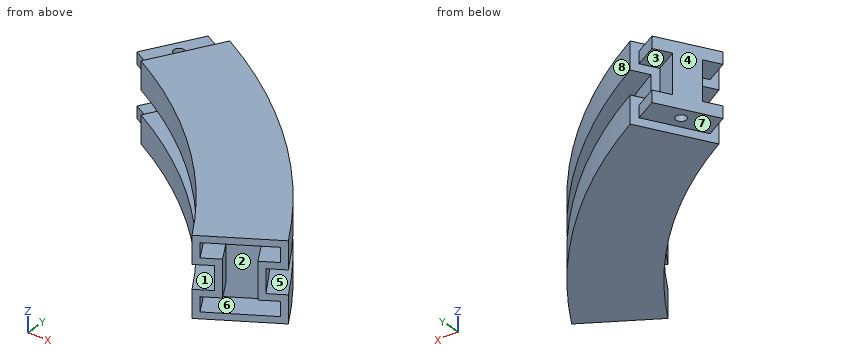
Autodesk Inventor part; units mm, degrees
ref_plane "Work Plane1" through (0, 50, 0) normal (0, 1, 0) x (-1, 0, 0)
ref_plane "Work Plane2" through (0, 0, -79) normal (0, 0, 1) x (1, 0, 0)
ref_plane "Work Plane3" through (-40, 45, 40) normal (0, -1, 0) x (1, 0, 0)
sketch "Sketch2" plane through (0, 0, 0) normal (0, 1, 0) x (-1, 0, 0)
  line L0 (15, 15) -> (-15, 15)
  line L1 (-15, -15) -> (15, -15)
  line L2 (15, 4.5) -> (8, 4.5)
  line L3 (8, 4.5) -> (8, -4.5)
  line L4 (8, -4.5) -> (15, -4.5)
  line L5 (-15, 4.5) -> (-8, 4.5)
  line L6 (-8, 4.5) -> (-8, -4.5)
  line L7 (-8, -4.5) -> (-15, -4.5)
  line L8 (15, -15) -> (15, -4.5)
  line L9 (15, 4.5) -> (15, 15)
  line L10 (-15, 15) -> (-15, 4.5)
  line L11 (-15, -4.5) -> (-15, -15)
  point P0 (0, 0)
  dimension "d18" = 9
  dimension "d19" = 7
  dimension "d21" = 16
  dimension "d22" = 30
  dimension "d23" = 15
  dimension "d24" = 4.5
  dimension "d25" = 8
sketch "Sketch6" plane through (0, 0, 0) normal (0, 0, 1) x (1, 0, 0)
  arc A0 (0, 0) -> (-110, 190.5256) centre (-220, 0) ccw
  line L0 (-220, 0) -> (-110, 190.5256) construction
  line L1 (-220, 0) -> (0, 0) construction
  dimension "d41" = 220
  dimension "d42" = 60
  dimension "d43" = 220
  dimension "d44" = 0
sweep "Sweep2" add profiles "Sketch2" path "Sketch6"
sketch "Sketch7" plane through (-102.5, 203.516, 4.5) normal (-0.8660254, 0.5, 0) x (0, 0, 1)
  line L0 (-16.5, -3) -> (-12, -3)
  line L1 (-12, -3) -> (-12, -10)
  line L2 (-12, -10) -> (3, -10)
  line L3 (3, -10) -> (3, -3)
  line L4 (3, -3) -> (7.5, -3)
  line L5 (7.5, -3) -> (7.5, -27)
  line L6 (7.5, -27) -> (3, -27)
  line L7 (3, -27) -> (3, -20)
  line L8 (3, -20) -> (-12, -20)
  line L9 (-12, -20) -> (-12, -27)
  line L10 (-12, -27) -> (-16.5, -27)
  line L11 (-16.5, -27) -> (-16.5, -3)
  line L12 (-19.5, 0) -> (-19.5, -30)
  line L13 (-9, -7) -> (-9, 0)
  line L14 (0, 0) -> (0, -7)
  line L15 (10.5, -30) -> (10.5, 0)
  line L16 (-19.5, -30) -> (-9, -30)
  line L17 (-9, 0) -> (-19.5, 0)
  line L18 (0, -30) -> (10.5, -30)
  line L19 (-9, -23) -> (0, -23)
  line L20 (0, -7) -> (-9, -7)
  point P0 (-4.5, -125)
  point P1 (-14.25, 0)
  dimension "d47" = 3
  dimension "d48" = 3
  dimension "d49" = 3
  dimension "d50" = 3
  dimension "d51" = 3
  dimension "d52" = 3
  dimension "d53" = 3
  dimension "d54" = 3
  dimension "d55" = 3
extrude "Extrusion3" add sketch "Sketch7" along normal blind 10
sketch "Sketch8" plane through (-116, 180.1333, -12) normal (0, 0, -1) x (-0.8660254, 0.5, 0)
  circle A0 centre (5, 12) radius 2
  line L0 (0, 0) -> (10, 0)
  line L1 (10, 24) -> (10, 0)
  point P0 (-190.5256, -98)
  dimension "d58" = 4
  dimension "d59" = 12
  dimension "d60" = 5
extrude "Extrusion4" cut sketch "Sketch8" against normal through all
sketch "Sketch9" plane through (0, 0, 0) normal (0, 1, 0) x (-1, 0, 0)
  line L0 (-40, 40) -> (40, 40)
  line L1 (40, 40) -> (40, -40)
  line L2 (40, -40) -> (-40, -40)
  line L3 (-40, -40) -> (-40, 40)
  point P0 (0, 0)
  dimension "d63" = 80
  dimension "d64" = 80
  dimension "d65" = 40
  dimension "d66" = 40
ref_plane "Work Plane1" through (0, 50, 0) normal (0, 1, 0) x (-1, 0, 0)
sketch "Sketch10" plane through (0, 50, 0) normal (0, 1, 0) x (-1, 0, 0)
  line L0 (-9.6, 15) -> (21.4, 15)
  line L1 (21.4, 15) -> (21.4, -15)
  line L2 (21.4, -15) -> (-9.6, -15)
  line L3 (-9.6, -15) -> (-9.6, 15)
  point P0 (0, 0)
  dimension "d68" = 30
  dimension "d69" = 9.6
  dimension "d70" = 15
  dimension "d71" = 31
loft "Loft1" add profiles "Sketch9", "Sketch10"
ref_plane "Work Plane2" through (0, 0, -79) normal (0, 0, 1) x (1, 0, 0)
sketch "Sketch11" plane through (0, 0, -79) normal (0, 0, 1) x (1, 0, 0)
  line L0 (50, -5) -> (-129.034, -5)
  line L1 (-129.034, -5) -> (-129.034, 135)
  line L2 (-129.034, 135) -> (-90, 202.6089)
  line L3 (-90, 202.6089) -> (50, 95)
  line L4 (50, -5) -> (50, 95)
  point P0 (0, 0)
  dimension "d77" = 100
  dimension "d79" = 140
  dimension "d80" = 67.6089
  dimension "d81" = 140
  dimension "d82" = 150
  dimension "d83" = 50
  dimension "d86" = 5
extrude "Extrusion5" [suppressed]
sketch "Sketch12" plane through (-40, 0, 40) normal (0, -1, 0) x (1, 0, 0)
  line L0 (70, -70) -> (10, -70)
  line L1 (10, -70) -> (10, -10)
  line L2 (10, -10) -> (70, -10)
  line L3 (70, -10) -> (70, -70)
  line L4 (0, 0) -> (0, -80)
  line L5 (0, -80) -> (80, -80)
  line L6 (80, -80) -> (80, 0)
  line L7 (80, 0) -> (0, 0)
  point P0 (40, -40)
  dimension "d87" = 10
  dimension "d88" = 10
  dimension "d89" = 10
  dimension "d90" = 10
ref_plane "Work Plane3" through (-40, 45, 40) normal (0, -1, 0) x (1, 0, 0)
sketch "Sketch14" plane through (-40, 45, 40) normal (0, -1, 0) x (1, 0, 0)
  line L0 (40.5, -40.5) -> (39.5, -40.5)
  line L1 (39.5, -40.5) -> (39.5, -39.5)
  line L2 (39.5, -39.5) -> (40.5, -39.5)
  line L3 (40.5, -39.5) -> (40.5, -40.5)
  line L4 (80, 0) -> (0, 0)
  line L5 (0, 0) -> (0, -80)
  point P0 (40, -40)
  point P1 (0, -40)
  dimension "d95" = 1
  dimension "d96" = 1
  dimension "d97" = 39.5
  dimension "d98" = 39.5
loft "Loft2" cut profiles "Sketch12", "Sketch14" contours L0 L1 L2 L3 / all
ref_plane "Work Plane4" through (9.6, 50, -45) normal (0, 0, -1) x (-1, 0, 0)
sketch "Sketch15" plane through (9.6, 50, -45) normal (0, 0, -1) x (-1, 0, 0)
  line L0 (-71.3683, -50) -> (104.0101, -50)
  line L1 (229.6, -50) -> (-99.4897, 140)
  line L2 (-99.4897, 140) -> (-99.4897, -50)
  line L3 (-99.4897, -50) -> (-71.3683, -50)
  line L4 (229.6, -50) -> (104.0101, -50)
  point P0 (9.6, -50)
  dimension "d104" = 220
  dimension "d105" = 30
  dimension "d107" = 190
extrude "Extrusion6" cut sketch "Sketch15" against normal through all
sketch "Sketch16" plane through (-42.4648, 102.5, -15) normal (0.5, -0.8660254, 0) x (0.8660254, 0.5, 0)
  line L0 (27.5, 27.5) -> (27.5, 22)
  line L1 (27.5, 22) -> (20.5, 22)
  line L2 (20.5, 22) -> (20.5, 8)
  line L3 (23, 10.5) -> (-7.5462, 10.5)
  line L4 (20.5, 8) -> (27.5, 8)
  line L5 (27.5, 8) -> (27.5, 2.5)
  line L6 (27.5, 2.5) -> (2.5, 2.5)
  line L7 (2.5, 2.5) -> (2.5, 8)
  line L8 (2.5, 8) -> (9.5, 8)
  line L9 (9.5, 8) -> (9.5, 22)
  line L10 (9.5, 22) -> (2.5, 22)
  line L11 (2.5, 27.5) -> (27.5, 27.5)
  line L12 (2.5, 22) -> (2.5, 27.5)
  line L13 (0, 30) -> (30, 30)
  line L14 (0, 19.5) -> (0, 30)
  line L15 (7, 19.5) -> (0, 19.5)
  line L16 (7, 10.5) -> (7, 19.5)
  line L17 (30, 0) -> (0, 0)
  line L18 (30, 10.5) -> (30, 0)
  line L19 (23, 19.5) -> (23, 10.5)
  point P0 (-14.4744, 15)
  dimension "d110" = 2.5
  dimension "d111" = 2.5
  dimension "d112" = 2.5
  dimension "d113" = 2.5
  dimension "d114" = 2.5
  dimension "d115" = 2.5
  dimension "d116" = 2.5
  dimension "d117" = 2.5
extrude "Extrusion7" cut sketch "Sketch16" against normal blind 10
properties part number "LightRail_endSection"
Source: CAD feature listing. Evaluate the final solid. Frame: model axes, mm. Face numbers are marked on the shaded views. A direction names the side the tool comes from. Round coordinates to 2 decimals unless told otherwise and drop trailing zeros. Order: outer loops, then holes, each group sorted by start corner. A loop starts at its lowest first (then second) coordinate and runs counter-clockwise, first axis right, second up. Notation, with made-up numbers: (70, 44.5) -> (111, 44.5) arc R10 cw to (111, 48.5) -> close; hole circle Ø1 at (5.5, -32.75). An arc over 180 degrees is marked (long way). One line per item, written item: value. Start each with the question number.
Q1. Section query D-D (z = 8.75). Return the cut outline in (x, y).
Q2. Section query B-B (y = 135). Return the cut outline in (x, z), plus the area to 3 significant figures.
Q3. Section query A-A (z = -3). Return the cut outline in (x, y), plus the area to 3 significant figures.
Q4. Access query for the marked faces 1, 2, 3, 4 and 5. Directions: +Z, -Z, +X, -X, +Y, -Y. A direction counts if a zero-diameter tool reaches every point of the face in a straight line with its end or side. Return the directions, or none.
Q5. Draft query along Z for the marked faces 6, 7 and 8. Return one class per face: pulls with the +Z half, pulls with the -Z half, needs draft (parallel to the pull), parting line crosses it, or undercut.
Q6. Pin query (flat end, axial travel): pin 1 (12 mm diameter, centred on x = -71, z = -8.5, fed in from +Y); pin 2 (3.5 mm diameter, centred on x = -118, y = 185, fed in from -Z); pin 3 (6 mm diameter, centred on y = 125.5, z = 10, fed in from -X). Return the tip coordinate at first contact, or that it passes through.
Q7. Material intervals for probe 1 along Z at (x, y) = (-71.5, 177); probe 2 along Y at (x, z) = (-115, 1.25); probe 3 along X at (y, z) = (194.5, -4.25), sorted ascending.
Q8. Section query C-C (x = -61). Return the cut outline in (y, z), plus the area to 3 significant figures.
Findings below:
1. outline: (-124.66, 185.13) -> (-116, 180.13) -> (-117.5, 177.54) arc R205 cw to (-42.46, 102.5) -> (-40.3, 103.75) -> (-45.3, 112.41) -> (-23.65, 124.91) -> (-18.65, 116.25) -> (-16.48, 117.5) arc R235 ccw to (-102.5, 203.52) -> (-104, 200.92) -> (-112.66, 205.92) -> close; hole circle Ø4 at (-114.33, 193.03)
2. outline: (-65.73, -15) -> (-27.65, -15) -> (-27.65, -4.5) -> (-36.26, -4.5) -> (-36.26, 4.5) -> (-27.65, 4.5) -> (-27.65, 15) -> (-65.73, 15) -> (-65.73, 4.5) -> (-56.54, 4.5) -> (-56.54, -4.5) -> (-65.73, -4.5) -> close
2. area: 982 mm²
3. outline: (-121.16, 191.2) -> (-112.5, 186.2) -> (-114, 183.6) arc R212 cw to (-36.4, 106) -> (-34.24, 107.25) -> (-39.24, 115.91) -> (-29.71, 121.41) -> (-24.71, 112.75) -> (-22.55, 114) arc R228 ccw to (-106, 197.45) -> (-107.5, 194.86) -> (-116.16, 199.86) -> close; hole circle Ø4 at (-114.33, 193.03)
3. area: 1,820 mm²
4. face 1: -X, -Y
4. face 2: none
4. face 3: +Y
4. face 4: +Z, -Z, -X, +Y
4. face 5: +X, +Y
5. face 6: undercut
5. face 7: pulls with the -Z half
5. face 8: needs draft
6. pin 1: y = 186.48
6. pin 2: z = -12
6. pin 3: x = -60.27
7. probe 1: -15 to -4.5, 4.5 to 15
7. probe 2: 187.64 to 191.14, 194.91 to 199.19
7. probe 3: -119.25 to -115.68, -112.98 to -101.03
8. outline: (129.4, -15) -> (173.04, -15) -> (173.04, -4.5) -> (163.41, -4.5) -> (163.41, 4.5) -> (173.04, 4.5) -> (173.04, 15) -> (129.4, 15) -> (129.4, 4.5) -> (140.22, 4.5) -> (140.22, -4.5) -> (129.4, -4.5) -> close
8. area: 1,130 mm²
